from build123d import *

# Parameters (mm, degrees)
F2_R          = 5
F3_DEPTH      = 5.501
F4_W          = 2
F4_H          = 9
F5_DEPTH      = 12
F5_DEPTH_BACK = 25
F6_R          = 1
F7_DEPTH      = 20


# Not quite as in the source:
# - a fillet or chamfer that OpenCascade refuses, or shapes differently, is made with other operations: its cross-section is extruded or revolved along the edge and cut away or added


with BuildPart() as f1:
    # F0 (on Front) → F1 (revolve)
    with BuildSketch(Plane.XZ):
        with BuildLine():
            Line((0, 5), (0, 5.5))
            ThreePointArc((0, 5.5), (-3.8890872965, 3.8890872965), (-5.5, 0))
            ThreePointArc((-5.5, 0), (-3.8890872965, -3.8890872965), (0, -5.5))
            Line((0, -5.5), (0, -5))
            ThreePointArc((0, -5), (-5, 0), (0, 5))
        make_face()
        with BuildLine():
            Line((0, -70.5), (0, -5.5))
            ThreePointArc((0, -5.5), (-3.8890872965, -3.8890872965), (-5.5, 0))
            Line((-5.5, 0), (-5.5, -70.5))
            Line((-5.5, -70.5), (0, -70.5))
        make_face()
    revolve(axis=Axis((0, 0, -32.5), (0, 0, -1)))

    # F2 (on Right) → F3 (cut, through all)
    with BuildSketch(Plane.YZ):
        Circle(F2_R)
    extrude(amount=-F3_DEPTH, mode=Mode.SUBTRACT)

    # F4 (on Right) → F5 (cut, two sides)
    with BuildSketch(Plane.YZ) as f5_sk:
        with Locations((0, 2.7013579383)):
            Rectangle(F4_W, F4_H)
    extrude(amount=-F5_DEPTH, mode=Mode.SUBTRACT)
    extrude(f5_sk.sketch, amount=F5_DEPTH_BACK, mode=Mode.SUBTRACT)

    # F6 (on face) → F7 (cut)
    with BuildSketch(Plane(origin=(0, 0, -70.5), x_dir=(1, 0, 0), z_dir=(0, 0, -1))):
        Circle(F6_R)
    extrude(amount=-F7_DEPTH, mode=Mode.SUBTRACT)

    # F8: fillet of radius 5 on 1 edges, made by hand

    # F8_s1 → F8_t2 (revolve, cut)
    with BuildSketch(Plane.XZ):
        with BuildLine():
            ThreePointArc((-5.5, -65.5250628145), (-4.2080992435, -68.8791647807), (-1, -70.5))
            Line((-1, -70.5), (-5.5, -70.5))
            Line((-5.5, -70.5), (-5.5, -65.5250628145))
        make_face()
    revolve(axis=Axis((0, 0, -70.5), (0, 0, -1)), mode=Mode.SUBTRACT)


solid = f1.part
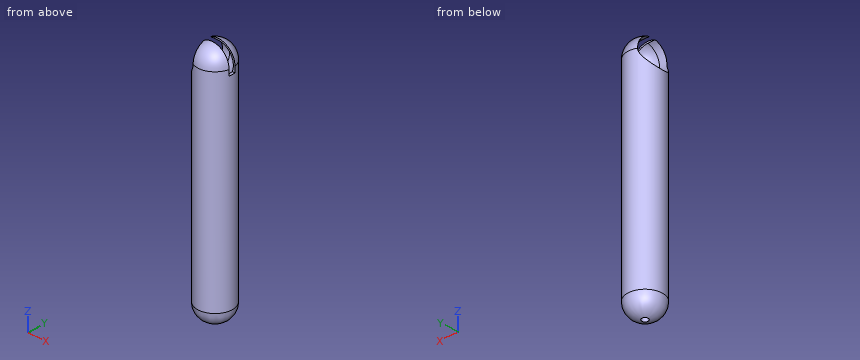
Read the model definition and answer for the solid it produces. Units are mm, in the model's axes. Coordinates: 2 decimals unless noted, no trailing zeros. Loops run counter-clockwise (first coordinate to the right, second up) from the corner with the lowest first, then second, coordinate; pieces in that order, holes last. Notation, with made-up numbers: (36, 89) -> (64, 89) arc R19 cw to (64, 122) -> close; hole circle Ø8 at (-18.5, -10). An arc over 180 degrees is marked (long way). Write item = value, one per line. Start each with the question number.
1) The part is cut by section A-A, the plane z = -60. Determine the outline of the cut face in (x, y).
2) Find the intervals of material crossed by L1, parallel to X at y = 0, z = -63.75; L2, parallel to Z at x = -1.75, y = -2.25, in increasing order. Write a range as from..to.
3) The part is cut by section B-B, the plane z = -26.5. Determine the outline of the cut face in (x, y).
4) Given P1, Ø0.8, axis at x = 5, y = 0, coming from the +Z side; P2, Ø2, axis at x = 3.5, z = 0, coming from the -Y side; P3, Ø5, axis at y = -3, z = -61, coming from the -X side, each flat-ended and moving along its own axis, determine where each tip first touches the part or whether it passes through.
Result:
q1.outline = circle Ø11 at (0, 0); hole circle Ø2 at (0, 0)
q2.L1 = -5.5..-1, 1..5.5
q2.L2 = -69.94..-4.47, 4.47..4.7
q3.outline = circle Ø11 at (0, 0)
q4.P1 = -1.8
q4.P2 = -4.9
q4.P3 = -5.48
